For this review, take the finished solid that the model builds, in its own axes (mm). Coordinates: 2 decimals unless noted, no trailing zeros. Write each loop counter-clockwise with the first axis right and the second up, starting at its lowest first coordinate (ties: lowest second). Pieces come first, ordered by that corner, then holes.
```python
from build123d import *

# Parameters (mm, degrees)
F1_DEPTH      = 2
F1_DEPTH_BACK = 2


with BuildPart() as f1:
    # F0 (on Front) → F1 (new body, two sides)
    with BuildSketch(Plane.XZ) as f1_sk:
        with BuildLine():
            Line((0, 10.7), (0, 12.7))
            ThreePointArc((0, 12.7), (-8.980256, 8.980256), (-12.7, 0))
            Line((-12.7, 0), (-10.7, 0))
            ThreePointArc((-10.7, 0), (-7.566043, 7.566043), (0, 10.7))
        make_face()
    extrude(amount=F1_DEPTH)
    extrude(f1_sk.sketch, amount=-F1_DEPTH_BACK)

    # F2: F1 across face


with BuildPart() as f1_1:
    add(f1.part)
    add(f1.part.mirror(Plane(origin=(0, 0, 11.7), x_dir=(0, 1, 0), z_dir=(1, 0, 0))))


solid = f1_1.part
```
1) Consider section B-B (y = 0.25). Give the boundary of the cut face in (x, z), then the cut area to 3 significant figures.
2) Clearance check with flat-ended pins moving along their axes: P1, Ø1.5, axis at y = 1.5, z = 7, coming from the +X side; P2, Ø1, axis at y = 1.5, z = 4, coming from the +X side. State where each tip first meets the part, or that it passes through.
3) Consider section D-D (x = 5.5). Give the boundary of the cut face in (y, z).
4) For L1, parallel to X at y = 0.15, z = 3.5; L2, parallel to X at y = -1.75, z = 5.75; L3, parallel to Z at x = -5.5, y = -0.6, list the stretches that pass through material, from the lowest coordinate up.
5) Consider section C-C (z = 1.5). Give the boundary of the cut face in (x, y), then the cut area to 3 significant figures.
6) Consider section A-A (z = 7.5). Give the boundary of the cut face in (x, y), then the cut area to 3 significant figures.
Results:
1. outline: (-12.7, 0) - (-10.7, 0) arc R10.7 cw to (0, 10.7) arc R10.7 cw to (10.7, 0) - (12.7, 0) arc R12.7 ccw to start
1. area: 73.5 mm2
2. P1: stops at x = 11.06
2. P2: stops at x = 12.21
3. outline: (-2, 9.18) - (2, 9.18) - (2, 11.45) - (-2, 11.45) - close
4. L1: x = -12.21 to -10.11, 10.11 to 12.21
4. L2: x = -11.32 to -9.02, 9.02 to 11.32
4. L3: z = 9.18 to 11.45
5. outline: (-12.61, -2) - (-10.59, -2) - (-10.59, 2) - (-12.61, 2) - close; (10.59, -2) - (12.61, -2) - (12.61, 2) - (10.59, 2) - close
5. area: 16.1 mm2
6. outline: (-10.25, -2) - (-7.63, -2) - (-7.63, 2) - (-10.25, 2) - close; (7.63, -2) - (10.25, -2) - (10.25, 2) - (7.63, 2) - close
6. area: 20.9 mm2
